```python
from build123d import *

# Parameters (mm, degrees)
BOSS_EXTRUDE1_DEPTH = 30
SKETCH2_R           = 0.615
CUT_EXTRUDE1_DEPTH  = 3


with BuildPart() as part:
    # Sketch1 → Boss-Extrude1 (new body)
    with BuildSketch(Plane.XY):
        Polygon((0, 0), (3, 0), (3, -3), (8, -3), (8, 0), (10, 0), (10, -4), (0, -4), align=None)
    extrude(amount=BOSS_EXTRUDE1_DEPTH)

    # Sketch2 → Cut-Extrude1 (cut)
    with BuildSketch(Plane.ZY):
        with Locations((3, -2)):
            Circle(SKETCH2_R)
        with Locations((6, -2)):
            Circle(SKETCH2_R)
        with Locations((24, -2)):
            Circle(SKETCH2_R)
        with Locations((27, -2)):
            Circle(SKETCH2_R)
    extrude(amount=-CUT_EXTRUDE1_DEPTH, mode=Mode.SUBTRACT)


solid = part.part
```
Geometry: final body of the model. Coordinates: model frame, mm. A direction names the side the tool comes from. Round coordinates to 2 decimals unless told otherwise and drop trailing zeros. Write each loop counter-clockwise with the first axis right and the second up, starting at its lowest first coordinate (ties: lowest second). Pieces come first, ordered by that corner, then holes.
Item 1: Section query C-C (z = 8.25). Return loops of the section in (x, y).
Item 2: Pin query (flat end, axial travel): P1, Ø1.5, axis at x = 5.5, z = 7.5, coming from the +Y side. Return the tip coordinate at first contact, or that it passes through.
Item 3: Section query A-A (y = -0.65). Return loops of the section in (x, z).
Item 4: Section query B-B (z = 24). Return loops of the section in (x, y) (3 decimals), plus the area to 3 significant figures.
Item 5: Set-up query: faces 1 (the face through (1.479, -1.973, 23.386)), 2 (the face through (5, -3, 15)), 3 (the face through (5.1, -3.3, 0)). Return all of +Z, -Z, +X, -X, +Y, -Y with unobstructed straight access to the full face (end or side cutting, diameter ignored); none if empty.
Item 6: Mould query, pull axis Y, two halves, no side actions, for faces 4 (the face through (8, -2, 15)), 5 (the face through (1.479, -1.973, 26.386)), 6 (the face through (1.479, -2.236, 6.568)), 7 (the face through (1, 0, 15)). Classes: +Y half, -Y half, draft (parallel to the pull), parting line (faces both ways), or undercut.
Item 7: Material intervals for L1, parallel to X at y = -0.7, z = 20.5; L2, parallel to Y at x = 1.6, z = 3 (3 decimals); L3, parallel to X at y = -2.2, z = 3.5, sorted ascending.
Completed:
1. outline: (0, -4) - (10, -4) - (10, 0) - (8, 0) - (8, -3) - (3, -3) - (3, 0) - (0, 0) - close
2. P1: stops at y = -3
3. outline: (0, 0) - (3, 0) - (3, 30) - (0, 30) - close; (8, 0) - (10, 0) - (10, 30) - (8, 30) - close
4. outline: (0, -4) - (10, -4) - (10, 0) - (8, 0) - (8, -3) - (3, -3) - (3, -2.615) - (0, -2.615) - close; (0, -1.385) - (3, -1.385) - (3, 0) - (0, 0) - close
4. area: 21.3 mm2
5. face 1: -X
5. face 2: +Z, -Z, +Y
5. face 3: -Z, +X, -X, +Y, -Y
6. face 4: draft
6. face 5: undercut
6. face 6: undercut
6. face 7: +Y half
7. L1: x = 0 to 3, 8 to 10
7. L2: y = -4 to -2.615, -1.385 to 0
7. L3: x = 8 to 10
